Geometry: final body of the model. Coordinates: model frame, mm. A direction names the side the tool comes from. Coordinates: 2 decimals unless noted, no trailing zeros. Loops run counter-clockwise (first coordinate to the right, second up) from the corner with the lowest first, then second, coordinate; pieces in that order, holes last. Notation, with made-up numbers: (-9, -15) -> (20, -15) arc R3 ccw to (20, -11) -> close; hole circle Ø2 at (25, 40.5). An arc over 180 degrees is marked (long way). One line per item, written item: value. Start each with the question number.
Item 1: Mould query, pull axis X, two halves, no side actions, for faces 4 (the cylindrical face through (9.75, 5.009, -4.223)), 5 (the flat face through (84, 8, -25.4)), 6 (the cylindrical face through (6.279, 5.009, -22.787)), 7 (the flat face through (13.97, 8, -4)). Classes: +X half, -X half, draft (parallel to the pull), parting line (faces both ways), or undercut.
Item 2: Section query D-D on x = 30. Return loops of the section in (y, z), then the cut area to 3 significant figures.
Item 3: Section query A-A on z = -16.51. Return loops of the section in (x, y) (3 decimals), then the cut area to 3 significant figures.
Item 4: Section query C-C on y = 3.5. Return loops of the section in (x, z) (3 decimals).
Item 5: Section query B-B on x = 7.62. Return loops of the section in (y, z).
Item 6: Contact query for flat-ended pins moving along their axis: pin 1 Ø1.9 at (x, y) = (100.5, 9) entering from -Z; pin 2 Ø3 at (y, z) = (8.5, -4.5) entering from +X; pin 3 Ø5 at (x, z) = (113.5, -4.5) entering from +Y. Output: stop coordinate, or through.
Item 7: Set-up query: faces 1 (the flat face through (13.97, 8, -29)), 2 (the cylindrical face through (0.724, 5.151, -0.764)), 3 (the cylindrical face through (151.676, 8.282, -8.384)). Return all of +Z, -Z, +X, -X, +Y, -Y with unobstructed straight access to the full face (end or side cutting, diameter ignored); none if empty.
Item 8: Ray query, probe 1 along X at (y, z) = (3.5, -16.51) (3 decimals); probe 2 along X at (y, z) = (3.75, -26.02); probe 3 along X at (y, z) = (0.5, -18). Return the intervals inside material, ascending. Write a range as from..to.
from build123d import *

# Parameters (mm, degrees)
SKETCH1_W           = 152.4
SKETCH1_H           = 33.02
SKETCH1_R           = 3.5
SKETCH1_R_2         = 3.175
BOSS_EXTRUDE1_DEPTH = 10.16
SKETCH3_W           = 7.62
SKETCH3_H           = 3.81
CUT_EXTRUDE1_DEPTH  = 138.43
FILLET1_R           = 2.54


with BuildPart() as part:
    # Sketch1 → Boss-Extrude1 (new body)
    with BuildSketch(Plane(origin=(0, 0, 0), x_dir=(1, 0, 0), z_dir=(0, 1, 0))):
        with Locations((76.2, 16.51)):
            Rectangle(SKETCH1_W, SKETCH1_H)
        with Locations(Location((7.62, 26.02, 0), (0, 0, 270))):
            Circle(SKETCH1_R, mode=Mode.SUBTRACT)
        with Locations(Location((7.62, 7, 0), (0, 0, 90))):
            Circle(SKETCH1_R, mode=Mode.SUBTRACT)
        with Locations(Location((130.8199949, 16.51, 0), (0, 0, 270))):
            Circle(SKETCH1_R_2, mode=Mode.SUBTRACT)
        with Locations(Location((36.8200051, 16.51, 0), (0, 0, 270))):
            Circle(SKETCH1_R_2, mode=Mode.SUBTRACT)
    extrude(amount=BOSS_EXTRUDE1_DEPTH)

    # Sketch3 → Cut-Extrude1 (cut)
    with BuildSketch(Plane(origin=(152.4, 0, 0), x_dir=(0, 0, -1), z_dir=(1, 0, 0))):
        with Locations((3.81, 8.255)):
            Rectangle(SKETCH3_W, SKETCH3_H)
        with Locations((29.21, 8.255)):
            Rectangle(SKETCH3_W, SKETCH3_H)
    extrude(amount=-CUT_EXTRUDE1_DEPTH, mode=Mode.SUBTRACT)

    # Fillet1
    fillet1_edges = [part.edges().sort_by_distance(p)[0] for p in [
        (152.4, 3.175, -33.02),
        (152.4, 3.175, 0),
        (13.97, 8.255, 0),
        (13.97, 8.255, -7.62),
        (152.4, 8.255, -7.62),
        (13.97, 8.255, -33.02),
        (13.97, 8.255, -25.4),
        (152.4, 8.255, -25.4),
        (0, 5.08, 0),
        (0, 5.08, -33.02),
    ]]
    fillet(fillet1_edges, radius=FILLET1_R)


solid = part.part
Reply:
1. face 4: undercut
1. face 5: draft
1. face 6: undercut
1. face 7: +X half
2. outline: (0, -33.02) -> (6.35, -33.02) -> (6.35, -25.4) -> (10.16, -25.4) -> (10.16, -7.62) -> (6.35, -7.62) -> (6.35, 0) -> (0, 0) -> close
2. area: 277 mm²
3. outline: (0, 0) -> (33.645, 0) -> (33.645, 10.16) -> (0, 10.16) -> close; (39.995, 0) -> (127.645, 0) -> (127.645, 10.16) -> (39.995, 10.16) -> close; (133.995, 0) -> (152.4, 0) -> (152.4, 10.16) -> (133.995, 10.16) -> close
3. area: 1,420 mm²
4. outline: (0, -30.48) arc R2.54 ccw to (2.54, -33.02) -> (149.86, -33.02) arc R2.54 ccw to (152.4, -30.48) -> (152.4, -2.54) arc R2.54 ccw to (149.86, 0) -> (2.54, 0) arc R2.54 ccw to (0, -2.54) -> close; hole circle Ø7 at (7.62, -26.02); hole circle Ø7 at (7.62, -7); hole circle Ø6.35 at (36.82, -16.51); hole circle Ø6.35 at (130.82, -16.51)
5. outline: (0, -33.02) -> (10.16, -33.02) -> (10.16, -29.52) -> (0, -29.52) -> close; (0, -22.52) -> (10.16, -22.52) -> (10.16, -10.5) -> (0, -10.5) -> close; (0, -3.5) -> (10.16, -3.5) -> (10.16, 0) -> (0, 0) -> close
6. pin 1: stops at z = -25.4
6. pin 2: stops at x = 14.14
6. pin 3: stops at y = 6.35
7. face 1: -Z, +X, +Y
7. face 2: +Z, -X, +Y, -Y
7. face 3: +Z, +X, +Y
8. probe 1: x = 0..33.645, 39.995..127.645, 133.995..152.4
8. probe 2: x = 0..4.12, 11.12..152.4
8. probe 3: x = 0..34.02, 39.62..128.02, 133.62..152.4
